Check sheet for the modelled part. Datum: model origin and axes. Units: mm. A direction names the side the tool comes from. Give positions to 0.01 mm unless a question says otherwise; leave off trailing zeros. Order: outer loops, then holes, each group sorted by start corner. A loop starts at its lowest first (then second) coordinate and runs counter-clockwise, first axis right, second up. Notation, with made-up numbers: (-29, 86) -> (-7, 86) arc R33 ccw to (-7, 119) -> close; hole circle Ø5 at (82, 83). An arc over 180 degrees is marked (long way). Write each question's results on one line, items separated by ' | '.
Autodesk Inventor part; units mm, degrees
ref_plane "Work Plane1" through (0, 21.5, 0) normal (0, -1, 0) x (1, 0, 0)
ref_plane "YZ Plane" through (0, 0, 0) normal (1, 0, 0) x (0, 1, 0)
ref_plane "XZ Plane" through (0, 0, 0) normal (0, 1, 0) x (-1, 0, 0)
sketch "Sketch1" plane through (0, 0, 0) normal (0, 1, 0) x (-1, 0, 0)
  circle A0 centre (0, 0) radius 4
  dimension "d0" = 8
extrude "Extrusion1" add sketch "Sketch1" against normal mid plane 50
sketch "Sketch2" plane through (0, -25, 0) normal (0, -1, 0) x (1, 0, 0)
  circle A0 centre (0, 0) radius 4
  line L0 (-5.6, 0) -> (5.6, 0)
  line L1 (-1.5, -1.5) -> (1.5, -1.5)
  line L2 (1.5, -1.5) -> (1.5, 1.5)
  line L3 (1.5, 1.5) -> (-1.5, 1.5)
  line L4 (-1.5, 1.5) -> (-1.5, -1.5)
  dimension "d3" = 3
  dimension "d4" = 3
  dimension "d5" = 1.5
  dimension "d6" = 1.5
extrude "Extrusion2" add sketch "Sketch2" along normal blind 4 contours L2 L1 L4 L0 | L0 L4 L3 L2
fillet "Fillet1" radius 0.2 8 edges at (1.5, -27, 1.5) (-1.5, -27, 1.5) (1.5, -27, -1.5) (0, -29, -1.5) (-1.5, -29, 0) (0, -29, 1.5) (1.5, -29, 0) (-1.5, -27, -1.5)
sketch "Sketch3" plane through (0, 0, 0) normal (0, 0, 1) x (1, 0, 0)
  line L0 (0, -4.8) -> (0, 0)
  line L1 (2.8, 0) -> (2.8, -4.8)
  arc A0 (-0.35, -2.4) -> (3.15, -2.4) centre (1.4, -2.4) ccw
  line L2 (0, -2.4) -> (2.8, -2.4) construction
  line L3 (-4, -25) -> (-4, 25)
  line L4 (-4, 25) -> (4, 25)
  line L5 (4, 25) -> (4, -25)
  line L6 (4, -25) -> (1.5, -25)
  line L7 (1.5, -25) -> (1.5, -28.8)
  arc A1 (1.3, -29) -> (1.5, -28.8) centre (1.3, -28.8) ccw
  line L8 (1.3, -29) -> (-1.3, -29)
  arc A2 (-1.5, -28.8) -> (-1.3, -29) centre (-1.3, -28.8) ccw
  line L9 (-1.5, -28.8) -> (-1.5, -25)
  line L10 (-1.5, -25) -> (-4, -25)
  line L11 (-1.5, -26.9) -> (1.5, -26.9) construction
  arc A3 (-1.75, -26.9) -> (1.75, -26.9) centre (0, -26.9) ccw
  line L12 (1.5, -26.9) -> (2.2631, -26.9) construction
  line L13 (-1.5, -26.9) -> (-1.9787, -26.9) construction
  line L14 (-1.75, -26.9) -> (1.75, -26.9)
  point P0 (1.4, -2.4)
  dimension "d10" = 1.75
  dimension "d11" = 3.5
revolve "Revolution1" add sketch "Sketch3" angle 360 about axis through (1.5, -26.9, 0) along (1, 0, 0) contours L14 L7 A3 L9 | L9 A3 L14 | L14 A3 L7
mirror "Mirror1" about plane through (0, 0, 0) normal (0, 1, 0) of "Extrusion2", "Revolution1", "Fillet1"
chamfer "Chamfer2" distance 0.3 angle 45 2 edges at (4, -25, 0) (4, 25, 0)
ref_plane "Work Plane1" through (0, 21.5, 0) normal (0, -1, 0) x (1, 0, 0)
split_face "Split1"
split_face "Split2"
equation "\"d3\" = d4"
equation "\"d5\" = 0.5 * d4"
equation "\"d6\" = 0.5 * d4"
properties part number "463-02" material "Steel"
1. Mould release check, pull along Y, two halves, no side actions. Record for faces 4 (the flat face through (0, 29, 0)), 5 (the flat face through (0, -29, 0)), 6 (the flat face through (1, 26, 1.5)): +Y half, -Y half, draft (parallel to the pull), parting line (faces both ways), or undercut.
Verdict:
face 4: +Y half | face 5: -Y half | face 6: undercut
2. Section check B-B on z = 0. Record the cut outline in (x, y), then the cut area to 3 significant figures.
Verdict:
outline: (-4, -24.7) -> (-3.7, -25) -> (-1.5, -25) -> (-1.5, -26) arc R1.75 ccw to (-1.5, -27.8) -> (-1.5, -28.8) arc R0.2 ccw to (-1.3, -29) -> (1.3, -29) arc R0.2 ccw to (1.5, -28.8) -> (1.5, -27.8) arc R1.75 ccw to (1.5, -26) -> (1.5, -25) -> (3.7, -25) -> (4, -24.7) -> (4, 24.7) -> (3.7, 25) -> (1.5, 25) -> (1.5, 26) arc R1.75 ccw to (1.5, 27.8) -> (1.5, 28.8) arc R0.2 ccw to (1.3, 29) -> (-1.3, 29) arc R0.2 ccw to (-1.5, 28.8) -> (-1.5, 27.8) arc R1.75 ccw to (-1.5, 26) -> (-1.5, 25) -> (-3.7, 25) -> (-4, 24.7) -> close | area: 425 mm^2
3. Section check A-A on x = 0. Record the cut outline in (y, z), then the cut area to 3 significant figures.
Verdict:
outline: (-29, -1.3) arc R0.2 ccw to (-28.8, -1.5) -> (-27.8, -1.5) arc R1.75 ccw to (-26, -1.5) -> (-25, -1.5) -> (-25, -3.7) -> (-24.7, -4) -> (24.7, -4) -> (25, -3.7) -> (25, -1.5) -> (26, -1.5) arc R1.75 ccw to (27.8, -1.5) -> (28.8, -1.5) arc R0.2 ccw to (29, -1.3) -> (29, 1.3) arc R0.2 ccw to (28.8, 1.5) -> (27.8, 1.5) arc R1.75 ccw to (26, 1.5) -> (25, 1.5) -> (25, 3.7) -> (24.7, 4) -> (-24.7, 4) -> (-25, 3.7) -> (-25, 1.5) -> (-26, 1.5) arc R1.75 ccw to (-27.8, 1.5) -> (-28.8, 1.5) arc R0.2 ccw to (-29, 1.3) -> close | area: 425 mm^2
4. Section check C-C on y = 21. Record the cut outline in (x, z), then the cut area to 3 significant figures.
Verdict:
outline: circle Ø8 at (0, 0) | area: 50.3 mm^2
5. Gauge pin test, flat ends, axial feed: pin 1 Ø0.8 at (y, z) = (-26.5, 0.5) entering from -X; pin 2 Ø2 at (x, y) = (-2.5, -21) entering from +Z; pin 3 Ø3 at (y, z) = (28, -0.5) entering from -X. Record the tip position at first contact, or that the pin passes through.
Verdict:
pin 1: stops at x = -1.73 | pin 2: stops at z = 3.71 | pin 3: stops at x = -1.75
6. Material ranges on probe 1 along Z at (x, y) = (-1.5, -22); probe 2 along Y at (x, z) = (1, 2.5); probe 3 along X at (y, z) = (10, -0.25), recorded low to high. Write a range as from..to.
Verdict:
probe 1: z = -3.71..3.71 | probe 2: y = -25..25 | probe 3: x = -3.99..3.99
7. Access from +Z, -Z, +X, -X, +Y, -Y to the whole of each face (thin tool, end or side, straight path). Record for faces 1 (the flat face through (1.5, 26, -1)), 2 (the flat face through (1, -26, 1.5)), 3 (the flat face through (-1, -26, -1.5)).
Verdict:
face 1: +X | face 2: +Z | face 3: -Z
